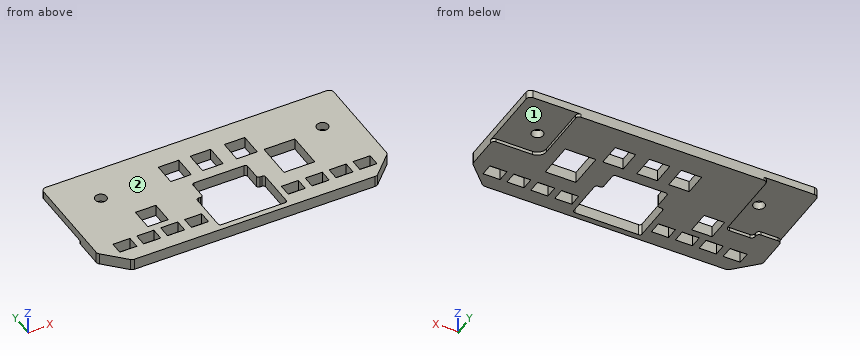
```python
from build123d import *

# Parameters (mm, degrees)
SKETCH1_W           = 18
SKETCH1_H           = 20
SKETCH1_W_2         = 27
SKETCH1_H_2         = 32
BOSS_EXTRUDE1_DEPTH = 10
SKETCH2_W           = 15
SKETCH2_H           = 11
CUT_EXTRUDE1_DEPTH  = 10
CUT_EXTRUDE2_DEPTH  = 3
FILLET1_R           = 3
FILLET2_R           = 3
FILLET3_R           = 3
FILLET4_R           = 3
FILLET5_R           = 3
CUT_EXTRUDE3_DEPTH  = 10
SKETCH5_R           = 5
CUT_EXTRUDE4_DEPTH  = 7


with BuildPart() as part:
    # Sketch1 → Boss-Extrude1 (new body)
    with BuildSketch(Plane.XY):
        with BuildLine():
            Line((-168.654215956, -33.412313616), (-150.997361707, -51.069167865))
            ThreePointArc((-150.997361707, -51.069167865), (-149.699668311, -51.936258871), (-148.168934582, -52.240740741))
            Line((-148.168934582, -52.240740741), (63.517356919, -52.240740741))
            ThreePointArc((63.517356919, -52.240740741), (65.048090649, -51.936258871), (66.345784044, -51.069167865))
            Line((66.345784044, -51.069167865), (84.002638293, -33.412313616))
            ThreePointArc((84.002638293, -33.412313616), (84.869729299, -32.114620221), (85.174211169, -30.583886491))
            Line((85.174211169, -30.583886491), (85.174211169, 53.759259259))
            ThreePointArc((85.174211169, 53.759259259), (84.002638293, 56.587686384), (81.174211169, 57.759259259))
            Line((81.174211169, 57.759259259), (-165.825788831, 57.759259259))
            ThreePointArc((-165.825788831, 57.759259259), (-168.654215956, 56.587686384), (-169.825788831, 53.759259259))
            Line((-169.825788831, 53.759259259), (-169.825788831, -30.583886491))
            ThreePointArc((-169.825788831, -30.583886491), (-169.521306961, -32.114620221), (-168.654215956, -33.412313616))
        make_face()
        with Locations((-68.825788831, 27.759259259)):
            Rectangle(SKETCH1_W, SKETCH1_H, mode=Mode.SUBTRACT)
        with Locations((-40.825788831, 27.759259259)):
            Rectangle(SKETCH1_W, SKETCH1_H, mode=Mode.SUBTRACT)
        with Locations((-10.825788831, 27.759259259)):
            Rectangle(SKETCH1_W, SKETCH1_H, mode=Mode.SUBTRACT)
        with Locations((-110.825788831, -12.240740741)):
            Rectangle(SKETCH1_W, SKETCH1_H, mode=Mode.SUBTRACT)
        with Locations((17.674211169, 1.759259259)):
            Rectangle(SKETCH1_W_2, SKETCH1_H_2, mode=Mode.SUBTRACT)
    extrude(amount=BOSS_EXTRUDE1_DEPTH)

    # Sketch2 → Cut-Extrude1 (cut)
    with BuildSketch(Plane.XY.offset(10)):
        with Locations((-146.325788831, -33.740740741)):
            Rectangle(SKETCH2_W, SKETCH2_H)
        with Locations((-125.325788831, -33.740740741)):
            Rectangle(SKETCH2_W, SKETCH2_H)
        with Locations((-104.325788831, -33.740740741)):
            Rectangle(SKETCH2_W, SKETCH2_H)
        with Locations((-83.325788831, -33.740740741)):
            Rectangle(SKETCH2_W, SKETCH2_H)
        with Locations((1.674211169, -33.740740741)):
            Rectangle(SKETCH2_W, SKETCH2_H)
        with Locations((22.674211169, -33.740740741)):
            Rectangle(SKETCH2_W, SKETCH2_H)
        with Locations((43.674211169, -33.740740741)):
            Rectangle(SKETCH2_W, SKETCH2_H)
        with Locations((64.674211169, -33.740740741)):
            Rectangle(SKETCH2_W, SKETCH2_H)
    extrude(amount=-CUT_EXTRUDE1_DEPTH, mode=Mode.SUBTRACT)

    # Sketch3 → Cut-Extrude2 (cut)
    with BuildSketch(Plane(origin=(0, 0, 0), x_dir=(-1, 0, 0), z_dir=(0, 0, -1))):
        with BuildLine():
            Line((-42.174211169, 57.759259259), (-85.174211169, 57.759259259))
            Line((-85.174211169, 57.759259259), (-85.174211169, -0.240740741))
            Line((-85.174211169, -0.240740741), (-50.174211169, -0.240740741))
            ThreePointArc((-50.174211169, -0.240740741), (-44.517356919, 2.10240501), (-42.174211169, 7.759259259))
            Line((-42.174211169, 7.759259259), (-42.174211169, 57.759259259))
        make_face()
        with BuildLine():
            Line((124.825788831, 57.759259259), (169.825788831, 57.759259259))
            Line((169.825788831, 57.759259259), (169.825788831, -2.240740741))
            Line((169.825788831, -2.240740741), (148.825788831, -2.240740741))
            Line((148.825788831, -2.240740741), (148.825788831, -6.240740741))
            ThreePointArc((148.825788831, -6.240740741), (147.947109175, -8.362061084), (145.825788831, -9.240740741))
            Line((145.825788831, -9.240740741), (127.825788831, -9.240740741))
            ThreePointArc((127.825788831, -9.240740741), (125.704468488, -8.362061084), (124.825788831, -6.240740741))
            Line((124.825788831, -6.240740741), (124.825788831, -1.240740741))
            Line((124.825788831, -1.240740741), (124.825788831, 57.759259259))
        make_face()
    extrude(amount=-CUT_EXTRUDE2_DEPTH, mode=Mode.SUBTRACT)

    # Fillet1
    fillet1_edges = [part.edges().sort_by_distance(p)[0] for p in [
        (-148.825788831, -2.240740741, 1.5),
    ]]
    fillet(fillet1_edges, radius=FILLET1_R)

    # Fillet2
    fillet2_edges = [part.edges().sort_by_distance(p)[0] for p in [
        (-169.825788831, -2.240740741, 1.5),
    ]]
    fillet(fillet2_edges, radius=FILLET2_R)

    # Fillet3
    fillet3_edges = [part.edges().sort_by_distance(p)[0] for p in [
        (-124.825788831, 57.759259259, 1.5),
    ]]
    fillet(fillet3_edges, radius=FILLET3_R)

    # Fillet4
    fillet4_edges = [part.edges().sort_by_distance(p)[0] for p in [
        (42.174211169, 57.759259259, 1.5),
    ]]
    fillet(fillet4_edges, radius=FILLET4_R)

    # Fillet5
    fillet5_edges = [part.edges().sort_by_distance(p)[0] for p in [
        (85.174211169, -0.240740741, 1.5),
    ]]
    fillet(fillet5_edges, radius=FILLET5_R)

    # Sketch4 → Cut-Extrude3 (cut)
    with BuildSketch(Plane(origin=(0, 0, 0), x_dir=(-1, 0, 0), z_dir=(0, 0, -1))):
        with BuildLine():
            Line((68.825788831, -47.240740741), (12.825788831, -47.240740741))
            ThreePointArc((12.825788831, -47.240740741), (11.411575269, -46.654954303), (10.825788831, -45.240740741))
            Line((10.825788831, -45.240740741), (10.825788831, -12.240740741))
            ThreePointArc((10.825788831, -12.240740741), (11.411575269, -10.826527178), (12.825788831, -10.240740741))
            Line((12.825788831, -10.240740741), (14.825788831, -10.240740741))
            ThreePointArc((14.825788831, -10.240740741), (16.240002394, -9.654954303), (16.825788831, -8.240740741))
            Line((16.825788831, -8.240740741), (16.825788831, 5.759259259))
            ThreePointArc((16.825788831, 5.759259259), (17.411575269, 7.173472822), (18.825788831, 7.759259259))
            Line((18.825788831, 7.759259259), (62.825788831, 7.759259259))
            ThreePointArc((62.825788831, 7.759259259), (64.240002394, 7.173472822), (64.825788831, 5.759259259))
            Line((64.825788831, 5.759259259), (64.825788831, -8.240740741))
            ThreePointArc((64.825788831, -8.240740741), (65.411575269, -9.654954303), (66.825788831, -10.240740741))
            Line((66.825788831, -10.240740741), (68.825788831, -10.240740741))
            ThreePointArc((68.825788831, -10.240740741), (70.240002394, -10.826527178), (70.825788831, -12.240740741))
            Line((70.825788831, -12.240740741), (70.825788831, -45.240740741))
            ThreePointArc((70.825788831, -45.240740741), (70.240002394, -46.654954303), (68.825788831, -47.240740741))
        make_face()
    extrude(amount=-CUT_EXTRUDE3_DEPTH, mode=Mode.SUBTRACT)

    # Sketch5 → Cut-Extrude4 (cut)
    with BuildSketch(Plane(origin=(0, 0, 3), x_dir=(-1, 0, 0), z_dir=(0, 0, -1))):
        with Locations((-57.174211169, 20.759259259)):
            Circle(SKETCH5_R)
        with Locations((134.825788831, 25.759259259)):
            Circle(SKETCH5_R)
    extrude(amount=-CUT_EXTRUDE4_DEPTH, mode=Mode.SUBTRACT)


solid = part.part
```
Geometry check sheet. Reference: the model listing, model coordinates, mm. Face numbers are marked on the shaded views. A direction names the side the tool comes from. Round coordinates to 2 decimals unless told otherwise and drop trailing zeros. Order: outer loops, then holes, each group sorted by start corner. A loop starts at its lowest first (then second) coordinate and runs counter-clockwise, first axis right, second up. Notation, with made-up numbers: (-39.5, 55) - (7.5, 55) arc R21 cw to (7.5, 72) - close; hole circle Ø7 at (-1, 49.25). An arc over 180 degrees is marked (long way). Use a Markdown table: item, result. Add a question column.
1) Section check D-D (y = 41). Record the cut outline in (x, z), then the cut area to 3 significant figures.
2) Section check C-C (x = -108). Record the cut outline in (y, z), then the cut area to 3 significant figures.
3) Section check B-B (y = -18.5). Record the cut outline in (x, z).
4) Set-up check for the marked faces 1 and 2: record each of +Z, -Z, +X, -X, +Y, -Y from which the full face is reachable in a straight line by a thin tool's end or side.
5) Gauge pin test, flat ends, axial feed: P1, Ø3, axis at y = -36, z = 5.5, coming from the +X side; P2, Ø5, axis at y = -36.5, z = 3, coming from the +X side. Record the tip position at first contact, or that the pin passes through.
6) Thickness scan on line 1 along Y through (x, z) = (7, 5.75); line 2 along Y through (x, z) = (-41.5, 1); line 3 along X through (y, z) = (35, 4). Record the ranges inside material, lowest first.
7) Section check A-A (x = -27.5). Record the cut outline in (y, z).
Established:
| question | item | result |
|---|---|---|
| 1 | outline | (-169.83, 3) - (-124.83, 3) - (-124.83, 0) - (42.17, 0) - (42.17, 3) - (85.17, 3) - (85.17, 10) - (-169.83, 10) - close |
| 1 | area | 2,290 mm2 |
| 2 | outline | (-52.24, 0) - (-39.24, 0) - (-39.24, 10) - (-52.24, 10) - close; (-28.24, 0) - (-22.24, 0) - (-22.24, 10) - (-28.24, 10) - close; (-2.24, 0) - (57.76, 0) - (57.76, 10) - (-2.24, 10) - close |
| 2 | area | 790 mm2 |
| 3 | outline | (-169.83, 0) - (-119.83, 0) - (-119.83, 10) - (-169.83, 10) - close; (-101.83, 0) - (-70.83, 0) - (-70.83, 10) - (-101.83, 10) - close; (-10.83, 0) - (85.17, 0) - (85.17, 10) - (-10.83, 10) - close |
| 4 | face 1 | -Z, +X, +Y |
| 4 | face 2 | +Z, +X, -X, +Y, -Y |
| 5 | P1 | x = 82.91 |
| 5 | P2 | x = 83.41 |
| 6 | line 1 | -52.24 to -39.24, -28.24 to -14.24, 17.76 to 57.76 |
| 6 | line 2 | -52.24 to -47.24, 7.76 to 17.76, 37.76 to 57.76 |
| 6 | line 3 | -169.83 to -77.83, -59.83 to -49.83, -31.83 to -19.83, -1.83 to 85.17 |
| 7 | outline | (-52.24, 0) - (-47.24, 0) - (-47.24, 10) - (-52.24, 10) - close; (7.76, 0) - (57.76, 0) - (57.76, 10) - (7.76, 10) - close |
